Autodesk Inventor part; units mm, degrees
ref_plane "YZ Plane" through (0, 0, 0) normal (1, 0, 0) x (0, 1, 0)
ref_plane "XZ Plane" through (0, 0, 0) normal (0, 1, 0) x (-1, 0, 0)
ref_plane "XY Plane" through (0, 0, 0) normal (0, 0, 1) x (1, 0, 0)
sketch "Skizze1" plane through (0, 0, 0) normal (1, 0, 0) x (0, 1, 0)
  line L0 (0, 1) -> (0, -3.6)
  line L1 (0, 1) -> (-3, 1)
  line L2 (-3, 1) -> (-3, 0)
  line L3 (-3, 0) -> (-2.1, 0)
  line L4 (-2.1, 0) -> (-2.1, -3.6)
  line L5 (-2.1, -3.6) -> (0, -3.6)
  point P0 (0, 0)
  dimension "d0" = 6
  dimension "d1" = 4.2
  dimension "d2" = 1
  dimension "Länge" = 3.6
revolve "Umdrehung1" add sketch "Skizze1" angle 360 about axis through (0, 0, 1) along (0, 0, -1)
sketch "Skizze2" plane through (0, 0, 1) normal (0, 0, 1) x (1, 0, 0)
  point P0 (0, 0)
  point P1 (0, 0)
hole "Bohrung1" at (0, 0, 1) direction (0, 0, -1) diameter 2.459 end through all countersink diameter 3 countersink angle 90
properties part number "9775036360R" material "Stahl, geschmiedet"
Part model, mm, in its own coordinate system. Round coordinates to 2 decimals unless told otherwise and drop trailing zeros. Order: outer loops, then holes, each group sorted by start corner. A loop starts at its lowest first (then second) coordinate and runs counter-clockwise, first axis right, second up. Notation, with made-up numbers: M 15.5,-22 L 35.5,-22 A6 cw 35.5,-15 Z; hole C 2,16.25 d6. An arc over 180 degrees is marked long. Answer in a Markdown table with one row per item. Add a question column.
Q1. Pin check, flat tips, straight feed: pin 1 (1 mm diameter, centred on x = -1.5, z = -1, fed in from -Y); pin 2 (1.5 mm diameter, centred on y = -1.5, z = -2.5, fed in from -X). Stop position of each tip, or through.
Q2. Cut at C-C on z = -1.8. Give the cut face in (x, y).
Q3. Cut at D-D on x = -2.4. Give the cut face in (y, z).
Q4. Mould opens along Y. For faces 1 (the face through (0.748, 0.976, -1.466)), 2 (the face through (2, -1.3, 0)), 3 (the face through (-0.631, -2.003, -1.825)) say: +Y half, -Y half, draft (parallel to the pull), parting line (faces both ways), or undercut.
Q5. Cut at A-A on y = 0. Give the cut face in (x, z), and give its area (3 significant figures).
Q6. Wall check: L1, parallel to Y at x = 0, z = -0.75; L2, parallel to Y at x = 0.55, z = -2.5. Give the ranges that are in metal, low to high. Write a range as from..to.
Established:
| question | item | result |
|---|---|---|
| 1 | pin 1 | stops at y = -1.85 |
| 1 | pin 2 | stops at x = -1.96 |
| 2 | outline | C 0,0 d4.2; hole C 0,0 d2.46 |
| 3 | outline | M -1.8,0 L 1.8,0 L 1.8,1 L -1.8,1 Z |
| 4 | face 1 | undercut |
| 4 | face 2 | draft |
| 4 | face 3 | parting line |
| 5 | outline | M -3,0 L -2.1,0 L -2.1,-3.6 L -1.23,-3.6 L -1.23,0.73 L -1.5,1 L -3,1 Z; M 1.23,-3.6 L 2.1,-3.6 L 2.1,0 L 3,0 L 3,1 L 1.5,1 L 1.23,0.73 Z |
| 5 | area | 9.74 mm2 |
| 6 | L1 | y = -2.1..-1.23, 1.23..2.1 |
| 6 | L2 | y = -2.03..-1.1, 1.1..2.03 |
